```python
from build123d import *

# Parameters (mm, degrees)
SKETCH6_R           = 134.318809958
EXTRUDE1_DEPTH      = 7.0358
SKETCH7_R           = 135.080809958
EXTRUDE2_DEPTH      = 21.6548
SKETCH8_R           = 134.318809958
EXTRUDE3_DEPTH      = 4.6188
SKETCH9_R           = 135.080809958
EXTRUDE4_DEPTH      = 733.4758
SKETCH10_R          = 134.318809958
EXTRUDE5_DEPTH      = 4.445
SKETCH11_R          = 135.080809958
EXTRUDE6_DEPTH      = 3.26898
SKETCH12_R          = 61.143546623
EXTRUDE7_DEPTH      = 31.20898
SKETCH13_W          = 86
SKETCH13_H          = 70
EXTRUDE8_DEPTH      = 106.29184
EXTRUDE9_DEPTH      = 7.07898
EXTRUDE9_DEPTH_BACK = 123.19
SKETCH15_R          = 69.240552209
EXTRUDE10_DEPTH     = 57.15
SKETCH16_R          = 31.191641703
CUT_EXTRUDE1_DEPTH  = 758.28398


with BuildPart() as part:
    # Sketch6 → Extrude1 (new body)
    with BuildSketch(Plane(origin=(0, 0, 0), x_dir=(1, 0, 0), z_dir=(0, 1, 0))):
        Circle(SKETCH6_R)
    extrude(amount=EXTRUDE1_DEPTH)

    # Sketch7 → Extrude2 (add)
    with BuildSketch(Plane(origin=(0, 7.0358, 0), x_dir=(-1, 0, 0), z_dir=(0, 1, 0))):
        Circle(SKETCH7_R)
    extrude(amount=EXTRUDE2_DEPTH)

    # Sketch8 → Extrude3 (add)
    with BuildSketch(Plane(origin=(0, 28.6906, 0), x_dir=(-1, 0, 0), z_dir=(0, 1, 0))):
        Circle(SKETCH8_R)
    extrude(amount=EXTRUDE3_DEPTH)

    # Sketch9 → Extrude4 (add)
    with BuildSketch(Plane(origin=(0, 33.3094, 0), x_dir=(-1, 0, 0), z_dir=(0, 1, 0))):
        Circle(SKETCH9_R)
    extrude(amount=EXTRUDE4_DEPTH)

    # Sketch10 → Extrude5 (add)
    with BuildSketch(Plane(origin=(0, 766.7852, 0), x_dir=(-1, 0, 0), z_dir=(0, 1, 0))):
        Circle(SKETCH10_R)
    extrude(amount=EXTRUDE5_DEPTH)

    # Sketch11 → Extrude6 (add)
    with BuildSketch(Plane(origin=(0, 771.2302, 0), x_dir=(-1, 0, 0), z_dir=(0, 1, 0))):
        Circle(SKETCH11_R)
    extrude(amount=EXTRUDE6_DEPTH)

    # Sketch12 → Extrude7 (add)
    with BuildSketch(Plane(origin=(0, 774.49918, 0), x_dir=(-1, 0, 0), z_dir=(0, 1, 0))):
        Circle(SKETCH12_R)
    extrude(amount=EXTRUDE7_DEPTH)

    # Sketch13 → Extrude8 (add)
    with BuildSketch(Plane(origin=(0, 805.70816, 0), x_dir=(-1, 0, 0), z_dir=(0, 1, 0))):
        with Locations((0, 4.8e-08)):
            Rectangle(SKETCH13_W, SKETCH13_H)
    extrude(amount=EXTRUDE8_DEPTH)

    # Sketch14 → Extrude9 (add, two sides)
    with BuildSketch(Plane.XY.offset(35.000000048)) as extrude9_sk:
        with BuildLine():
            Line((37.999996487, 886.888547526), (37.999996487, 851.111452474))
            ThreePointArc((37.999996487, 851.111452474), (-41.9999984, 869), (37.999996487, 886.888547526))
        make_face()
    extrude(amount=EXTRUDE9_DEPTH)
    extrude(extrude9_sk.sketch, amount=-EXTRUDE9_DEPTH_BACK)

    # Sketch15 → Extrude10 (add)
    with BuildSketch(Plane(origin=(0, 0, -88.189999952), x_dir=(-1, 0, 0), z_dir=(0, 0, -1))):
        with Locations((0, 869)):
            Circle(SKETCH15_R)
    extrude(amount=EXTRUDE10_DEPTH)

    # Sketch16 → Cut-Extrude1 (cut)
    with BuildSketch(Plane.XZ):
        Circle(SKETCH16_R)
    extrude(amount=-CUT_EXTRUDE1_DEPTH, mode=Mode.SUBTRACT)


solid = part.part
```
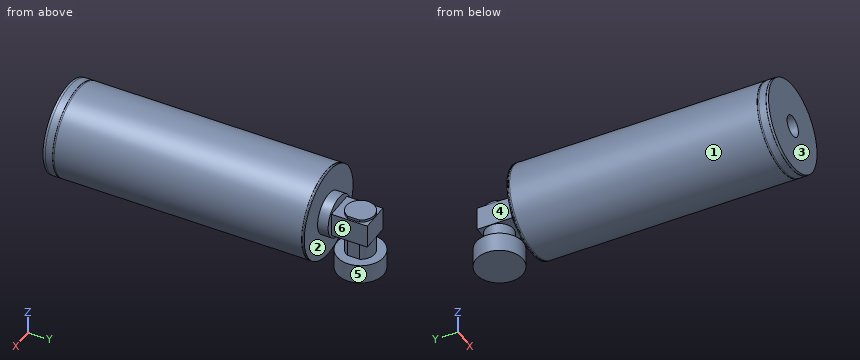
Here's how the part is built. I have some questions about the finished solid (model axes, mm). Face numbers are marked on the shaded views. A direction names the side the tool comes from. Coordinates: 2 decimals unless noted, no trailing zeros. Loops run counter-clockwise (first coordinate to the right, second up) from the corner with the lowest first, then second, coordinate; pieces in that order, holes last. Notation, with made-up numbers: (79, -38) -> (109, -38) arc R17 ccw to (109, -21) -> close; hole circle Ø9 at (-20, 18). An arc over 180 degrees is marked (long way). Return JSON: item names as keys, results as strings.
1) If we section it at C-C, the plane y = 712: Write out the boundary of the cut face in (x, z).
Results below:
{"outline": "circle Ø270.16 at (0, 0); hole circle Ø62.38 at (0, 0)"}
2) I need wall thicknesses on line 1 (Y direction, x = 4, z = -60.5); line 2 (Y direction, x = 79.5, z = -45.5); line 3 (Z direction, x = 0, y = 589). Which ranges of each line are inside material? Lowest first, please. Write a range as from..to.
Results below:
{"line 1": "0..805.71, 827.19..910.81", "line 2": "0..774.5", "line 3": "-135.08..-31.19, 31.19..135.08"}
3) If we section it at D-D, the plane x = 111: Write out the boundary of the cut face in (y, z), then the cut area to 3 significant figures.
Results below:
{"outline": "(0, -75.63) -> (7.04, -75.63) -> (7.04, -76.98) -> (28.69, -76.98) -> (28.69, -75.63) -> (33.31, -75.63) -> (33.31, -76.98) -> (766.79, -76.98) -> (766.79, -75.63) -> (771.23, -75.63) -> (771.23, -76.98) -> (774.5, -76.98) -> (774.5, 76.98) -> (771.23, 76.98) -> (771.23, 75.63) -> (766.79, 75.63) -> (766.79, 76.98) -> (33.31, 76.98) -> (33.31, 75.63) -> (28.69, 75.63) -> (28.69, 76.98) -> (7.04, 76.98) -> (7.04, 75.63) -> (0, 75.63) -> close", "area": "119,000 mm²"}
4) For the marked faces 4, 5 and 6, which set-ups out of +Z, -Z, +X, -X, +Y, -Y let a thin tool reach every point of the face, with its end or its side?
Results below:
{"face 4": "+Z, -X, +Y", "face 5": "-Z", "face 6": "+Z, +X, +Y"}
5) Thinking about a two-plate mould opening in Y: for the marked faces 1, 2 and 3, which applies, +Y half, -Y half, draft (parallel to the pull), parting line (faces both ways), or undercut?
Results below:
{"face 1": "draft", "face 2": "undercut", "face 3": "-Y half"}
6) If we section it at B-B, the plane y = 869: Write out the boundary of the cut face in (x, z), then the cut area to 3 significant figures.
Results below:
{"outline": "(-69.24, -145.34) -> (69.24, -145.34) -> (69.24, -88.19) -> (38, -88.19) -> (38, -35) -> (43, -35) -> (43, 35) -> (38, 35) -> (38, 42.08) -> (-42, 42.08) -> (-42, 35) -> (-43, 35) -> (-43, -35) -> (-42, -35) -> (-42, -88.19) -> (-69.24, -88.19) -> close", "area": "18,800 mm²"}
7) If we section it at A-A, the plane z = -122.5: Write out the boundary of the cut face in (x, y).
Results below:
{"outline": "circle Ø138.48 at (0, 869); (-56.93, 7.04) -> (-55.09, 7.04) -> (-55.09, 0) -> (55.09, 0) -> (55.09, 7.04) -> (56.93, 7.04) -> (56.93, 28.69) -> (55.09, 28.69) -> (55.09, 33.31) -> (56.93, 33.31) -> (56.93, 766.79) -> (55.09, 766.79) -> (55.09, 771.23) -> (56.93, 771.23) -> (56.93, 774.5) -> (-56.93, 774.5) -> (-56.93, 771.23) -> (-55.09, 771.23) -> (-55.09, 766.79) -> (-56.93, 766.79) -> (-56.93, 33.31) -> (-55.09, 33.31) -> (-55.09, 28.69) -> (-56.93, 28.69) -> close"}
8) Will these pins go through, and if not, where does the flat tip stop? pin 1 (10.5 mm diameter, centred on y = 874, z = -69.5, fed in from +X); pin 2 (12 mm diameter, centred on x = -28, y = 365.5, fed in from +Z); pin 3 (6 mm diameter, centred on x = 72, z = -13.5, fed in from +Y).
Results below:
{"pin 1": "x = 38", "pin 2": "z = 133.28", "pin 3": "y = 774.5"}
